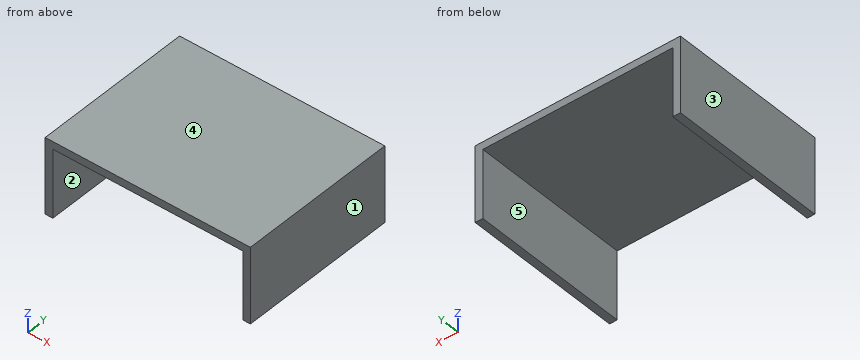
```python
from build123d import *

# Parameters (mm, degrees)
F0_W     = 2.54
F0_H     = 53.34
F0_W_2   = 58.42
F1_DEPTH = 25.4
F2_DEPTH = 22.86
F3_DEPTH = 22.86


with BuildPart() as f1:
    # F0 (on Top) → F1 (new body)
    with BuildSketch(Plane.XY):
        with Locations((-33.02, 0)):
            Rectangle(F0_W, F0_H)
        with Locations((-30.48, 0)):
            Rectangle(F0_W, F0_H)
        Rectangle(F0_W_2, F0_H)
        with Locations((30.48, 0)):
            Rectangle(F0_W, F0_H)
        with Locations((33.02, 0)):
            Rectangle(F0_W, F0_H)
    extrude(amount=F1_DEPTH)

    # F0 (on Top) → F2 (cut)
    with BuildSketch(Plane.XY):
        with Locations((-30.48, 0)):
            Rectangle(F0_W, F0_H)
        with Locations((30.48, 0)):
            Rectangle(F0_W, F0_H)
    extrude(amount=F2_DEPTH, mode=Mode.SUBTRACT)

    # F0 (on Top) → F3 (cut)
    with BuildSketch(Plane.XY):
        Rectangle(F0_W_2, F0_H)
    extrude(amount=F3_DEPTH, mode=Mode.SUBTRACT)


solid = f1.part
```
For this review, take the finished solid that the model builds, in its own axes (mm). Face numbers are marked on the shaded views. A direction names the side the tool comes from. Coordinates: 2 decimals unless noted, no trailing zeros. Loops run counter-clockwise (first coordinate to the right, second up) from the corner with the lowest first, then second, coordinate; pieces in that order, holes last. Notation, with made-up numbers: (19, -2) -> (24, -2) arc R20 ccw to (24, 13) -> close; hole circle Ø11 at (-39.75, -32). An arc over 180 degrees is marked (long way). Return JSON: item names as keys, results as strings. Group by question number.
(1) Consider section C-C, the plane x = -25. Give the boundary of the cut face in (y, z), plus the area to 3 significant figures.
(2) Consider section A-A, the plane z = 7.75. Give the boundary of the cut face in (x, y), plus the area to 3 significant figures.
(3) Consider section B-B, the plane y = -3.5. Give the boundary of the cut face in (x, z).
(4) Mouldability with a two-part tool opening along X and no side actions: class the marked faces 3, 4 and 5 as pulls with the +X half, pulls with the -X half, needs draft (parallel to the pull), parting line crosses it, or undercut.
(5) To check wall thickness, follow L1, parallel to X at y = 2.5, z = 5; L2, parallel to Z at x = -4, y = -14.5. State the ranges of each line that lie inside material, in increasing order.
(6) For pin 1 Ø4 at (x, y) = (-6.5, -3) entering from -Z, flat-tipped, find the tip position at first contact; note if it passes through.
(7) Tool access review of the marked faces 1 and 2: name each direction out of +Z, -Z, +X, -X, +Y, -Y from which nothing blocks a thin tool from reaching the whole face with its end or side.
Results below:
{
 "1": {"outline": "(-26.67, 22.86) -> (26.67, 22.86) -> (26.67, 25.4) -> (-26.67, 25.4) -> close", "area": "135 mm2"},
 "2": {"outline": "(-34.29, -26.67) -> (-31.75, -26.67) -> (-31.75, 26.67) -> (-34.29, 26.67) -> close; (31.75, -26.67) -> (34.29, -26.67) -> (34.29, 26.67) -> (31.75, 26.67) -> close", "area": "271 mm2"},
 "3": {"outline": "(-34.29, 0) -> (-31.75, 0) -> (-31.75, 22.86) -> (31.75, 22.86) -> (31.75, 0) -> (34.29, 0) -> (34.29, 25.4) -> (-34.29, 25.4) -> close"},
 "4": {"face 3": "pulls with the -X half", "face 4": "needs draft", "face 5": "undercut"},
 "5": {"L1": "x = -34.29 to -31.75, 31.75 to 34.29", "L2": "z = 22.86 to 25.4"},
 "6": {"pin 1": "stops at z = 22.86"},
 "7": {"face 1": "+Z, -Z, +X, +Y, -Y", "face 2": "-Z, +Y, -Y"}
}
